```python
from build123d import *

# Parameters (mm, degrees)
SKETCH1_R               = 13
SKETCH1_R_2             = 1.5
BOSS_EXTRUDE1_DEPTH     = 3
CUT_EXTRUDE1_REACH      = 39.336
CUT_EXTRUDE1_END_RADIUS = 19
SKETCH2_R               = 1.5


with BuildPart() as part:
    # Sketch1 → Boss-Extrude1 (new, symmetric)
    with BuildSketch(Plane.XY):
        with BuildLine():
            Line((-21.065374433, 6.5), (-32, 6.5))
            Line((-32, 6.5), (-32, -6.5))
            Line((-32, -6.5), (-21.065374433, -6.5))
            ThreePointArc((-21.065374433, -6.5), (-18.513822618, -7.20004845), (-16.676754759, -9.104166667))
            ThreePointArc((-16.676754759, -9.104166667), (19, 0), (-16.676754759, 9.104166667))
            ThreePointArc((-16.676754759, 9.104166667), (-18.513822618, 7.20004845), (-21.065374433, 6.5))
        make_face()
        Circle(SKETCH1_R, mode=Mode.SUBTRACT)
        with Locations((-26, 3.5)):
            Circle(SKETCH1_R_2, mode=Mode.SUBTRACT)
        with Locations(Location((-26, -3.5, 0), (0, 0, 180))):
            Circle(SKETCH1_R_2, mode=Mode.SUBTRACT)
    extrude(amount=BOSS_EXTRUDE1_DEPTH, both=True)

    # Cut-Extrude1: up to this cylinder (the profile starts inside it)
    cut_extrude1_end = Plane(origin=(0, 0, 0), z_dir=(0, 0, -1)) * Cylinder(CUT_EXTRUDE1_END_RADIUS, 117.672, mode=Mode.PRIVATE)
    # Sketch2 → Cut-Extrude1 (cut, up to the surface)
    with BuildSketch(Plane(origin=(0, 0, 0), x_dir=(1, 0, 0), z_dir=(0, 1, 0)), mode=Mode.PRIVATE) as cut_extrude1_sk1:
        with Locations(Location((0, 0, 0), (0, 0, 90))):
            Circle(SKETCH2_R)
    cut_extrude1_tool1 = extrude(cut_extrude1_sk1.sketch, amount=CUT_EXTRUDE1_REACH, mode=Mode.PRIVATE) & cut_extrude1_end
    add(cut_extrude1_tool1.solids().sort_by_distance((0, 0, 0))[0], mode=Mode.SUBTRACT)


solid = part.part
```
Work out the finished part from the listing and answer in its coordinate system (mm). A direction names the side the tool comes from. Coordinates: 2 decimals unless noted, no trailing zeros. Loops run counter-clockwise (first coordinate to the right, second up) from the corner with the lowest first, then second, coordinate; pieces in that order, holes last. Notation, with made-up numbers: M 53,22 L 97,22 A20 ccw 97,27 Z; hole C -3,-13 d8. An arc over 180 degrees is marked long. Use CSV: the item, a comma, the result in double quotes. Start each with the question number.
(1) Given pin 1 Ø5 at (x, y) = (-26, 3.5) entering from +Z; pin 2 Ø1 at (x, z) = (7.5, -2.5) entering from -Y, each flat-ended and moving along its own axis, determine where each tip first touches the part or whether it passes through.
(2) Find section A-A, the plane y = 0. Give the vertices of the cut face in (x, z).
(3) For a pull along Y with two mould halves and no side action, classify faces 1 (the face through (-24.5, -3.57, -0.04)), 2 (the face through (-27, -6.5, 0)), 3 (the face through (-0.45, 15.91, -1.43)) as +Y half, -Y half, draft (parallel to the pull), parting line (faces both ways), or undercut.
(4) Consider line 1 (Y direction, x = -26, z = -0.4); line 2 (X direction, y = -3.5, z = -1); line 3 (X direction, y = 3, z = -2). Determine where each line is inside the solid, lowest interval first.
(5) Find section D-D, the plane x = 6. Give the vertices of the cut face in (y, z).
(6) Find section B-B, the plane x = -26. Give the vertices of the cut face in (y, z), then the cut area to 3 significant figures.
(7) Find section C-C, the plane z = 0.5. Give the vertices of the cut face in (x, y).
(8) For faces 4 (the face through (-32, 0, 0)), 5 (the face through (-26, 6.5, 0)), determine the directions among +Z, -Z, +X, -X, +Y, -Y from which every point of the face is accessible in a straight line to the end or side of a thin tool.
Recorded:
1,pin 1,"stops at z = 3"
1,pin 2,"stops at y = -17.66"
2,outline,"M -32,-3 L -13,-3 L -13,3 L -32,3 Z; M 13,-3 L 19,-3 L 19,3 L 13,3 Z"
3,face 1,"undercut"
3,face 2,"-Y half"
3,face 3,"draft"
4,line 1,"y = -6.5 to -5, -2 to 2, 5 to 6.5"
4,line 2,"x = -32 to -27.5, -24.5 to -12.52, 12.52 to 18.67"
4,line 3,"x = -32 to -27.41, -24.59 to -12.65, 12.65 to 18.76"
5,outline,"M -18.03,-3 L -11.53,-3 L -11.53,3 L -18.03,3 Z; M 11.53,-3 L 18.03,-3 L 18.03,3 L 11.53,3 Z"
6,outline,"M -6.5,-3 L -5,-3 L -5,3 L -6.5,3 Z; M -2,-3 L 2,-3 L 2,3 L -2,3 Z; M 5,-3 L 6.5,-3 L 6.5,3 L 5,3 Z"
6,area,"42.0 mm^2"
7,outline,"M -32,-6.5 L -21.07,-6.5 A5 cw -16.68,-9.1 A19 ccw long 1.41,18.95 L 1.41,12.92 A13 cw long -1.41,12.92 L -1.41,18.95 A19 ccw -16.68,9.1 A5 cw -21.07,6.5 L -32,6.5 Z; hole C -26,-3.5 d3; hole C -26,3.5 d3"
8,face 4,"+Z, -Z, -X, +Y, -Y"
8,face 5,"+Z, -Z, -X, +Y"
